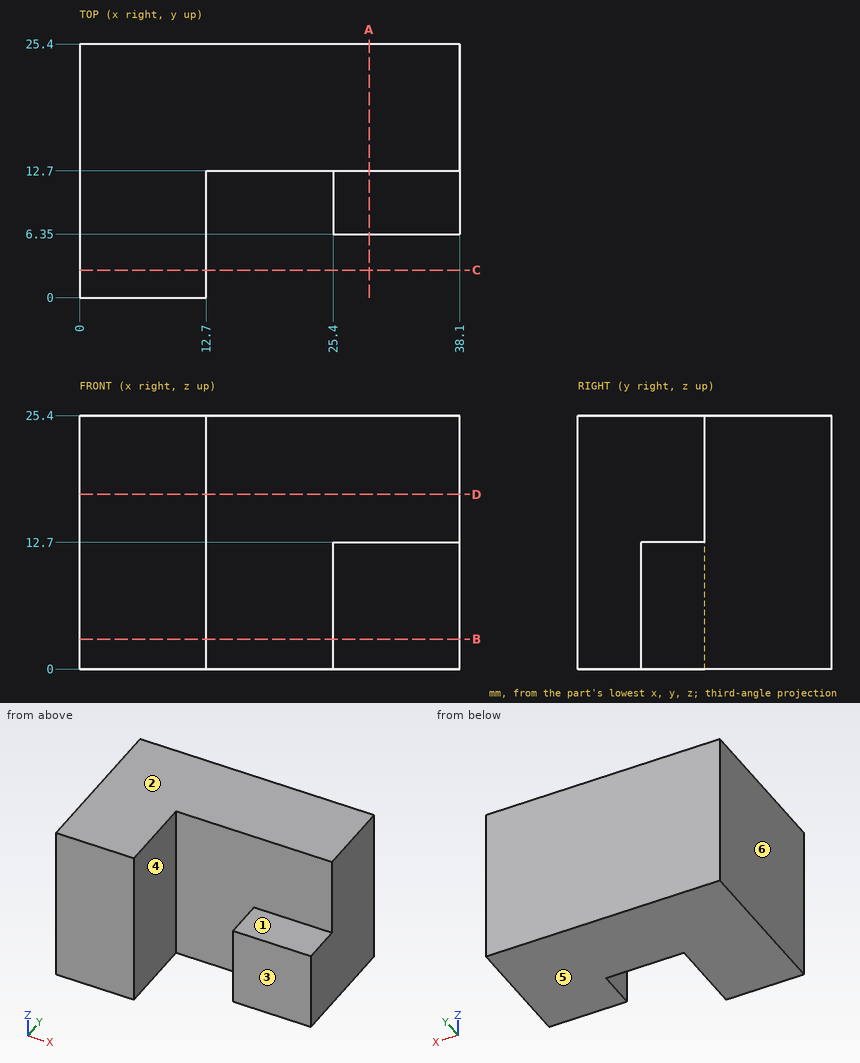
Part print with two shaded views. Sizes in mm from the minimum x, y, z corner. A direction names the side the tool comes from. Round coordinates to 2 decimals unless told otherwise and drop trailing zeros. Loops run counter-clockwise (first coordinate to the right, second up) from the corner with the lowest first, then second, coordinate; pieces in that order, holes last. Notation, with made-up numbers: M -34.75,65 L 11.25,65 A12 cw 11.25,79 Z; hole C 28,8.5 d4. An arc over 180 degrees is marked long. Return JSON: item names as keys, results as strings. Group by question number.
(1) Saw through at D-D, the plane z = 17.5. List the corners of the cut face in (x, y), and give its area (3 significant figures).
(2) Saw through at B-B, the plane z = 3. List the corners of the cut face in (x, y).
(3) Drop flat-ended pins along their axis: P1, Ø1.9, axis at x = 29, y = 10.5, coming from the +Z side; P2, Ø1, axis at y = 9.5, z = 17, coming from the -X side; P3, Ø10, axis at x = 29, z = 7, coming from the -Y side; P4, Ø4, axis at y = 7.5, z = 17, coming from the +X side. Give the stop position or say it passes through.
(4) Saw through at C-C, the plane y = 2.75. List the corners of the cut face in (x, z), and give its area (3 significant figures).
(5) Tool access for the marked faces 1, 2 and 3: list every direction of +Z, -Z, +X, -X, +Y, -Y with a clear straight run to the whole face (end or side of a thin tool).
(6) Wall check: probe 1 along X at (y, z) = (11.5, 5.75); probe 2 along Y at (x, z) = (13, 17.75); probe 3 along X at (y, z) = (8.75, 14.25). Give the ranges that are in metal, low to high. Write a range as [from, to].
(7) Saw through at A-A, the plane x = 29. List the corners of the cut face in (y, z), and give its area (3 significant figures).
(8) Mould opens along X. For the marked faces 4, 5 and 6 say: +X half, -X half, draft (parallel to the pull), parting line (faces both ways), or undercut.
Answer list:
{
 "1": {"outline": "M 0,0 L 12.7,0 L 12.7,12.7 L 38.1,12.7 L 38.1,25.4 L 0,25.4 Z", "area": "645 mm2"},
 "2": {"outline": "M 0,0 L 12.7,0 L 12.7,12.7 L 25.4,12.7 L 25.4,6.35 L 38.1,6.35 L 38.1,25.4 L 0,25.4 Z"},
 "3": {"P1": "z = 12.7", "P2": "x = 0", "P3": "y = 6.35", "P4": "x = 12.7"},
 "4": {"outline": "M 0,0 L 12.7,0 L 12.7,25.4 L 0,25.4 Z", "area": "323 mm2"},
 "5": {"face 1": "+Z, +X, -Y", "face 2": "+Z, +X, -X, +Y, -Y", "face 3": "+Z, -Z, +X, -Y"},
 "6": {"probe 1": "[0, 12.7], [25.4, 38.1]", "probe 2": "[12.7, 25.4]", "probe 3": "[0, 12.7]"},
 "7": {"outline": "M 6.35,0 L 25.4,0 L 25.4,25.4 L 12.7,25.4 L 12.7,12.7 L 6.35,12.7 Z", "area": "403 mm2"},
 "8": {"face 4": "undercut", "face 5": "draft", "face 6": "-X half"}
}
